Input: part model. Units: mm. Frame: model coordinates. Face numbers are marked on the shaded views. A direction names the side the tool comes from. Coordinates: 2 decimals unless noted, no trailing zeros. Order: outer loops, then holes, each group sorted by start corner. A loop starts at its lowest first (then second) coordinate and runs counter-clockwise, first axis right, second up. Notation, with made-up numbers: M 88,41.5 L 132,41.5 A18 ccw 132,61.5 Z; hole C -35,76 d7. An arc over 180 degrees is marked long. Answer in a Markdown table with one row per item.
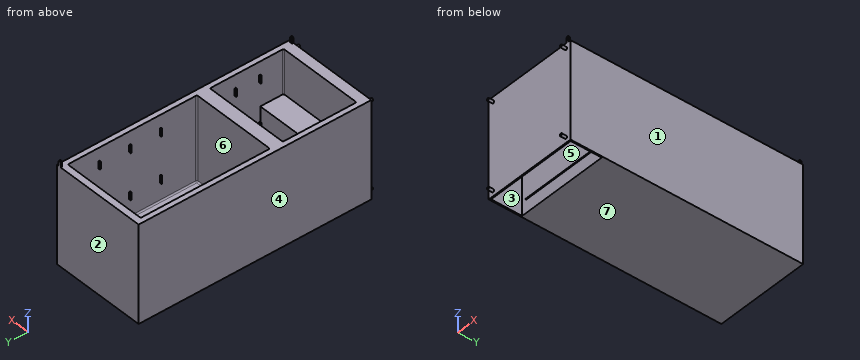
from build123d import *
from OCP.BRepFilletAPI import BRepFilletAPI_MakeChamfer

# Parameters (mm, degrees)
ESBO_O1_W                = 740
ESBO_O1_H                = 750
RESSALTO_EXTRUS_O1_DEPTH = 1800
ESBO_O5_W                = 660
ESBO_O5_H                = 1000
ESBO_O5_H_2              = 570
CORTE_EXTRUS_O1_DEPTH    = 650
FILETE1_R                = 10
ESBO_O7_R                = 10
RESSALTO_EXTRUS_O3_DEPTH = 40
ESBO_O10_W               = 55
ESBO_O10_H               = 10
RESSALTO_EXTRUS_O4_DEPTH = 15
ESBO_O14_W               = 55
ESBO_O14_H               = 10
RESSALTO_EXTRUS_O5_DEPTH = 15
CHANFRO1_SIZE            = 5
CHANFRO1_SIZE2           = 5.958767963
RESSALTO_EXTRUS_O6_DEPTH = 10
ESBO_O18_R               = 5
CORTE_EXTRUS_O2_DEPTH    = 5
ESBO_O19_W               = 720
ESBO_O19_H               = 240
CORTE_EXTRUS_O5_DEPTH    = 400
RESSALTO_EXTRUS_O8_REACH = 2073.835


with BuildPart() as part:
    # Esboço1 → Ressalto-extrusão1 (new body)
    with BuildSketch(Plane(origin=(0, 0, 0), x_dir=(1, 0, 0), z_dir=(0, 1, 0))):
        with Locations((370, 375)):
            Rectangle(ESBO_O1_W, ESBO_O1_H)
    extrude(amount=RESSALTO_EXTRUS_O1_DEPTH)

    # Esboço5 → Corte-extrusão1 (cut)
    with BuildSketch(Plane.XY):
        with Locations((370, 1250)):
            Rectangle(ESBO_O5_W, ESBO_O5_H)
        with Locations((370, 365)):
            Rectangle(ESBO_O5_W, ESBO_O5_H_2)
    extrude(amount=-CORTE_EXTRUS_O1_DEPTH, mode=Mode.SUBTRACT)

    # Filete1
    filete1_edges = [part.edges().sort_by_distance(p)[0] for p in [
        (40, 1250, -650),
        (40, 750, -325),
        (370, 1750, -650),
        (40, 1750, -325),
        (700, 1250, -650),
        (700, 1750, -325),
        (370, 750, -650),
        (700, 750, -325),
        (40, 365, -650),
        (40, 80, -325),
        (370, 650, -650),
        (40, 650, -325),
        (700, 365, -650),
        (700, 650, -325),
        (370, 80, -650),
        (700, 80, -325),
    ]]
    fillet(filete1_edges, radius=FILETE1_R)

    # Esboço7 → Ressalto-extrusão3 (add)
    with BuildSketch(Plane.XZ):
        with Locations(Location((40, -40, 0), (0, 0, 270))):
            Circle(ESBO_O7_R)
        with Locations(Location((700, -40, 0), (0, 0, 270))):
            Circle(ESBO_O7_R)
        with Locations(Location((700, -710, 0), (0, 0, 270))):
            Circle(ESBO_O7_R)
        with Locations(Location((40, -710, 0), (0, 0, 270))):
            Circle(ESBO_O7_R)
    extrude(amount=RESSALTO_EXTRUS_O3_DEPTH)

    # Esboço10 → Ressalto-extrusão4 (add)
    with BuildSketch(Plane(origin=(40, 0, 0), x_dir=(0, 0, -1), z_dir=(1, 0, 0))):
        with Locations((127.5, 1507.5)):
            Rectangle(ESBO_O10_W, ESBO_O10_H)
        with Locations((482.5, 1507.5)):
            Rectangle(ESBO_O10_W, ESBO_O10_H)
        with Locations((482.5, 1270)):
            Rectangle(ESBO_O10_W, ESBO_O10_H)
        with Locations((482.5, 1032.5)):
            Rectangle(ESBO_O10_W, ESBO_O10_H)
        with Locations((127.5, 1270)):
            Rectangle(ESBO_O10_W, ESBO_O10_H)
        with Locations((127.5, 1032.5)):
            Rectangle(ESBO_O10_W, ESBO_O10_H)
    ressalto_extrus_o4 = extrude(amount=RESSALTO_EXTRUS_O4_DEPTH)

    # Espelhar4: Ressalto-extrusão4 across plane
    add(ressalto_extrus_o4.mirror(Plane(origin=(370, 0, 0), x_dir=(0, 0, 1), z_dir=(1, 0, 0))))

    # Esboço14 → Ressalto-extrusão5 (add)
    with BuildSketch(Plane(origin=(40, 0, 0), x_dir=(0, 0, -1), z_dir=(1, 0, 0))):
        with Locations((127.5, 455)):
            Rectangle(ESBO_O14_W, ESBO_O14_H)
        with Locations((482.5, 455)):
            Rectangle(ESBO_O14_W, ESBO_O14_H)
        with Locations((482.5, 265)):
            Rectangle(ESBO_O14_W, ESBO_O14_H)
        with Locations((127.5, 265)):
            Rectangle(ESBO_O14_W, ESBO_O14_H)
    ressalto_extrus_o5 = extrude(amount=RESSALTO_EXTRUS_O5_DEPTH)

    # Espelhar5: Ressalto-extrusão5 across plane
    add(ressalto_extrus_o5.mirror(Plane(origin=(370, 0, 0), x_dir=(0, 0, 1), z_dir=(1, 0, 0))))

    # Chanfro1: one chamfer whose edges measure the first distance from different faces: ONE call of the kernel's chamfer builder (chamfer() names one face for all edges)
    chanfro1_edges_1 = [part.edges().sort_by_distance(p)[0] for p in [
        (55, 1502.5, -127.5),
    ]]
    chanfro1_side_1 = [part.faces().sort_by_distance(p)[0] for p in [
        (55, 1507.5, -127.5),
    ]]
    chanfro1_edges_2 = [part.edges().sort_by_distance(p)[0] for p in [
        (55, 1502.5, -482.5),
    ]]
    chanfro1_side_2 = [part.faces().sort_by_distance(p)[0] for p in [
        (55, 1507.5, -482.5),
    ]]
    chanfro1_edges_3 = [part.edges().sort_by_distance(p)[0] for p in [
        (55, 1265, -482.5),
    ]]
    chanfro1_side_3 = [part.faces().sort_by_distance(p)[0] for p in [
        (55, 1270, -482.5),
    ]]
    chanfro1_edges_4 = [part.edges().sort_by_distance(p)[0] for p in [
        (55, 1027.5, -482.5),
    ]]
    chanfro1_side_4 = [part.faces().sort_by_distance(p)[0] for p in [
        (55, 1032.5, -482.5),
    ]]
    chanfro1_edges_5 = [part.edges().sort_by_distance(p)[0] for p in [
        (55, 1265, -127.5),
    ]]
    chanfro1_side_5 = [part.faces().sort_by_distance(p)[0] for p in [
        (55, 1270, -127.5),
    ]]
    chanfro1_edges_6 = [part.edges().sort_by_distance(p)[0] for p in [
        (55, 1027.5, -127.5),
    ]]
    chanfro1_side_6 = [part.faces().sort_by_distance(p)[0] for p in [
        (55, 1032.5, -127.5),
    ]]
    chanfro1_edges_7 = [part.edges().sort_by_distance(p)[0] for p in [
        (685, 1502.5, -127.5),
    ]]
    chanfro1_side_7 = [part.faces().sort_by_distance(p)[0] for p in [
        (692.5, 1502.5, -127.5),
    ]]
    chanfro1_edges_8 = [part.edges().sort_by_distance(p)[0] for p in [
        (685, 1502.5, -482.5),
    ]]
    chanfro1_side_8 = [part.faces().sort_by_distance(p)[0] for p in [
        (692.5, 1502.5, -482.5),
    ]]
    chanfro1_edges_9 = [part.edges().sort_by_distance(p)[0] for p in [
        (685, 1265, -482.5),
    ]]
    chanfro1_side_9 = [part.faces().sort_by_distance(p)[0] for p in [
        (692.5, 1265, -482.5),
    ]]
    chanfro1_edges_10 = [part.edges().sort_by_distance(p)[0] for p in [
        (685, 1027.5, -482.5),
    ]]
    chanfro1_side_10 = [part.faces().sort_by_distance(p)[0] for p in [
        (692.5, 1027.5, -482.5),
    ]]
    chanfro1_edges_11 = [part.edges().sort_by_distance(p)[0] for p in [
        (685, 1265, -127.5),
    ]]
    chanfro1_side_11 = [part.faces().sort_by_distance(p)[0] for p in [
        (692.5, 1265, -127.5),
    ]]
    chanfro1_edges_12 = [part.edges().sort_by_distance(p)[0] for p in [
        (685, 1027.5, -127.5),
    ]]
    chanfro1_side_12 = [part.faces().sort_by_distance(p)[0] for p in [
        (692.5, 1027.5, -127.5),
    ]]
    chanfro1_edges_13 = [part.edges().sort_by_distance(p)[0] for p in [
        (55, 450, -127.5),
    ]]
    chanfro1_side_13 = [part.faces().sort_by_distance(p)[0] for p in [
        (55, 455, -127.5),
    ]]
    chanfro1_edges_14 = [part.edges().sort_by_distance(p)[0] for p in [
        (55, 450, -482.5),
    ]]
    chanfro1_side_14 = [part.faces().sort_by_distance(p)[0] for p in [
        (55, 455, -482.5),
    ]]
    chanfro1_edges_15 = [part.edges().sort_by_distance(p)[0] for p in [
        (55, 260, -482.5),
    ]]
    chanfro1_side_15 = [part.faces().sort_by_distance(p)[0] for p in [
        (55, 265, -482.5),
    ]]
    chanfro1_edges_16 = [part.edges().sort_by_distance(p)[0] for p in [
        (55, 260, -127.5),
    ]]
    chanfro1_side_16 = [part.faces().sort_by_distance(p)[0] for p in [
        (55, 265, -127.5),
    ]]
    chanfro1_edges_17 = [part.edges().sort_by_distance(p)[0] for p in [
        (685, 450, -127.5),
    ]]
    chanfro1_side_17 = [part.faces().sort_by_distance(p)[0] for p in [
        (692.5, 450, -127.5),
    ]]
    chanfro1_edges_18 = [part.edges().sort_by_distance(p)[0] for p in [
        (685, 450, -482.5),
    ]]
    chanfro1_side_18 = [part.faces().sort_by_distance(p)[0] for p in [
        (692.5, 450, -482.5),
    ]]
    chanfro1_edges_19 = [part.edges().sort_by_distance(p)[0] for p in [
        (685, 260, -482.5),
    ]]
    chanfro1_side_19 = [part.faces().sort_by_distance(p)[0] for p in [
        (692.5, 260, -482.5),
    ]]
    chanfro1_edges_20 = [part.edges().sort_by_distance(p)[0] for p in [
        (685, 260, -127.5),
    ]]
    chanfro1_side_20 = [part.faces().sort_by_distance(p)[0] for p in [
        (692.5, 260, -127.5),
    ]]
    chanfro1 = BRepFilletAPI_MakeChamfer(part.part.solid().wrapped)
    for e in chanfro1_edges_1:
        chanfro1.Add(CHANFRO1_SIZE, CHANFRO1_SIZE2, e.wrapped, chanfro1_side_1[0].wrapped)  # the first distance lies on this face
    for e in chanfro1_edges_2:
        chanfro1.Add(CHANFRO1_SIZE, CHANFRO1_SIZE2, e.wrapped, chanfro1_side_2[0].wrapped)  # the first distance lies on this face
    for e in chanfro1_edges_3:
        chanfro1.Add(CHANFRO1_SIZE, CHANFRO1_SIZE2, e.wrapped, chanfro1_side_3[0].wrapped)  # the first distance lies on this face
    for e in chanfro1_edges_4:
        chanfro1.Add(CHANFRO1_SIZE, CHANFRO1_SIZE2, e.wrapped, chanfro1_side_4[0].wrapped)  # the first distance lies on this face
    for e in chanfro1_edges_5:
        chanfro1.Add(CHANFRO1_SIZE, CHANFRO1_SIZE2, e.wrapped, chanfro1_side_5[0].wrapped)  # the first distance lies on this face
    for e in chanfro1_edges_6:
        chanfro1.Add(CHANFRO1_SIZE, CHANFRO1_SIZE2, e.wrapped, chanfro1_side_6[0].wrapped)  # the first distance lies on this face
    for e in chanfro1_edges_7:
        chanfro1.Add(CHANFRO1_SIZE, CHANFRO1_SIZE2, e.wrapped, chanfro1_side_7[0].wrapped)  # the first distance lies on this face
    for e in chanfro1_edges_8:
        chanfro1.Add(CHANFRO1_SIZE, CHANFRO1_SIZE2, e.wrapped, chanfro1_side_8[0].wrapped)  # the first distance lies on this face
    for e in chanfro1_edges_9:
        chanfro1.Add(CHANFRO1_SIZE, CHANFRO1_SIZE2, e.wrapped, chanfro1_side_9[0].wrapped)  # the first distance lies on this face
    for e in chanfro1_edges_10:
        chanfro1.Add(CHANFRO1_SIZE, CHANFRO1_SIZE2, e.wrapped, chanfro1_side_10[0].wrapped)  # the first distance lies on this face
    for e in chanfro1_edges_11:
        chanfro1.Add(CHANFRO1_SIZE, CHANFRO1_SIZE2, e.wrapped, chanfro1_side_11[0].wrapped)  # the first distance lies on this face
    for e in chanfro1_edges_12:
        chanfro1.Add(CHANFRO1_SIZE, CHANFRO1_SIZE2, e.wrapped, chanfro1_side_12[0].wrapped)  # the first distance lies on this face
    for e in chanfro1_edges_13:
        chanfro1.Add(CHANFRO1_SIZE, CHANFRO1_SIZE2, e.wrapped, chanfro1_side_13[0].wrapped)  # the first distance lies on this face
    for e in chanfro1_edges_14:
        chanfro1.Add(CHANFRO1_SIZE, CHANFRO1_SIZE2, e.wrapped, chanfro1_side_14[0].wrapped)  # the first distance lies on this face
    for e in chanfro1_edges_15:
        chanfro1.Add(CHANFRO1_SIZE, CHANFRO1_SIZE2, e.wrapped, chanfro1_side_15[0].wrapped)  # the first distance lies on this face
    for e in chanfro1_edges_16:
        chanfro1.Add(CHANFRO1_SIZE, CHANFRO1_SIZE2, e.wrapped, chanfro1_side_16[0].wrapped)  # the first distance lies on this face
    for e in chanfro1_edges_17:
        chanfro1.Add(CHANFRO1_SIZE, CHANFRO1_SIZE2, e.wrapped, chanfro1_side_17[0].wrapped)  # the first distance lies on this face
    for e in chanfro1_edges_18:
        chanfro1.Add(CHANFRO1_SIZE, CHANFRO1_SIZE2, e.wrapped, chanfro1_side_18[0].wrapped)  # the first distance lies on this face
    for e in chanfro1_edges_19:
        chanfro1.Add(CHANFRO1_SIZE, CHANFRO1_SIZE2, e.wrapped, chanfro1_side_19[0].wrapped)  # the first distance lies on this face
    for e in chanfro1_edges_20:
        chanfro1.Add(CHANFRO1_SIZE, CHANFRO1_SIZE2, e.wrapped, chanfro1_side_20[0].wrapped)  # the first distance lies on this face
    add(Compound.cast(chanfro1.Shape()), mode=Mode.REPLACE)

    # Esboço17 → Ressalto-extrusão6 (add)
    with BuildSketch(Plane(origin=(0, 1800, 0), x_dir=(1, 0, 0), z_dir=(0, 1, 0))):
        with BuildLine():
            Line((703.893019461, 0), (723.893019461, 0))
            Line((723.893019461, 0), (723.893019461, -35))
            ThreePointArc((723.893019461, -35), (713.893019461, -45), (703.893019461, -35))
            Line((703.893019461, -35), (703.893019461, 0))
        make_face()
    ressalto_extrus_o6 = extrude(amount=-RESSALTO_EXTRUS_O6_DEPTH)

    # Esboço18 → Corte-extrusão2 (cut)
    with BuildSketch(Plane.XZ.offset(-1790)):
        with Locations(Location((713.893019461, 35, 0), (0, 0, 270))):
            Circle(ESBO_O18_R)
    corte_extrus_o2 = extrude(amount=-CORTE_EXTRUS_O2_DEPTH, mode=Mode.SUBTRACT)

    # Espelhar6: Ressalto-extrusão6, Corte-extrusão2 across plane
    add(ressalto_extrus_o6.mirror(Plane.ZX.offset(900)))
    add(corte_extrus_o2.mirror(Plane.ZX.offset(900)), mode=Mode.SUBTRACT)

    # Esboço19 → Corte-extrusão5 (cut)
    with BuildSketch(Plane(origin=(0, 0, -750), x_dir=(-1, 0, 0), z_dir=(0, 0, -1))):
        with Locations((-370, 130)):
            Rectangle(ESBO_O19_W, ESBO_O19_H)
    extrude(amount=-CORTE_EXTRUS_O5_DEPTH, mode=Mode.SUBTRACT)

    # Esboço21 → Ressalto-extrusão8 (add, up to next)
    with BuildSketch(Plane.ZY.offset(-700), mode=Mode.PRIVATE) as ressalto_extrus_o8_sk1:
        Polygon((-640, 250), (-350, 250), (-350, 0), (-340, 0), (-340, 260), (-640, 260), align=None)
    ressalto_extrus_o8_tool1 = extrude(ressalto_extrus_o8_sk1.sketch, amount=RESSALTO_EXTRUS_O8_REACH, mode=Mode.PRIVATE) - part.part
    add(ressalto_extrus_o8_tool1.solids().sort_by_distance((700, 253.969887, -495))[0])


solid = part.part
1) Contact query for flat-ended pins moving along their axis: pin 1 (11 mm diameter, centred on x = 696, z = -131, fed in from -Y); pin 2 (8 mm diameter, centred on x = 50, y = 1506, fed in from +Z); pin 3 (3 mm diameter, centred on x = 368, y = 355, fed in from +Z). Output: stop coordinate, or through.
Resolved:
| item | result |
|---|---|
| pin 1 | stops at y = 0 |
| pin 2 | stops at z = -100 |
| pin 3 | stops at z = -650 |
2) Material intervals for probe 1 along Y at (x, z) = (180, -78); probe 2 along Y at (x, z) = (65.5, -596.5); probe 3 along X at (y, z) = (339, -89), sorted ascending.
Resolved:
| item | result |
|---|---|
| probe 1 | y = 0 to 80, 650 to 750, 1750 to 1800 |
| probe 2 | y = 0 to 10, 250 to 260, 650 to 750, 1750 to 1800 |
| probe 3 | x = 0 to 40, 700 to 740 |
3) Reachability of the marked faces 5, 6 and 7 from +Z, -Z, +X, -X, +Y, -Y: full face, straight path, thin tool, end or side. Return the list, or none.
Resolved:
| item | result |
|---|---|
| face 5 | -Z |
| face 6 | +Z |
| face 7 | -Z, +X, -X, +Y, -Y |
4) Mould query, pull axis X, two halves, no side actions, for the marked faces 1, 2, 3 and 4. Classes: +X half, -X half, draft (parallel to the pull), parting line (faces both ways), or undercut.
Resolved:
| item | result |
|---|---|
| face 1 | +X half |
| face 2 | draft |
| face 3 | undercut |
| face 4 | -X half |
5) Cut plane C-C, the plane z = -399. Output: boundary loops of the cut face in (x, y).
Resolved:
| item | result |
|---|---|
| outline | M 0,0 L 740,0 L 740,1800 L 0,1800 Z; hole M 10,10 L 730,10 L 730,250 L 10,250 Z; hole M 40,260 L 700,260 L 700,640 A10 ccw 690,650 L 50,650 A10 ccw 40,640 Z; hole M 40,760 A10 ccw 50,750 L 690,750 A10 ccw 700,760 L 700,1740 A10 ccw 690,1750 L 50,1750 A10 ccw 40,1740 Z |
6) Cut plane A-A, the plane x = 480. Output: boundary loops of the cut face in (y, z), and give its area (3 significant figures).
Resolved:
| item | result |
|---|---|
| outline | M 0,-750 L 10,-750 L 10,-350 L 250,-350 L 250,-640 L 260,-640 L 260,-340 L 80,-340 L 80,0 L 0,0 Z; M 250,-750 L 1800,-750 L 1800,0 L 1750,0 L 1750,-640 A10 cw 1740,-650 L 760,-650 A10 cw 750,-640 L 750,0 L 650,0 L 650,-640 A10 cw 640,-650 L 250,-650 Z |
| area | 289,000 mm2 |
7) Cut plane D-D, the plane y = 399.5. Output: boundary loops of the cut face in (x, z), and give its area (3 significant figures).
Resolved:
| item | result |
|---|---|
| outline | M 0,-750 L 740,-750 L 740,0 L 700,0 L 700,-640 A10 cw 690,-650 L 50,-650 A10 cw 40,-640 L 40,0 L 0,0 Z |
| area | 126,000 mm2 |
8) Cut plane B-B, the plane z = -218. Output: boundary loops of the cut face in (x, y), and give its area (3 significant figures).
Resolved:
| item | result |
|---|---|
| outline | M 0,0 L 740,0 L 740,1800 L 0,1800 Z; hole M 40,90 A10 ccw 50,80 L 690,80 A10 ccw 700,90 L 700,640 A10 ccw 690,650 L 50,650 A10 ccw 40,640 Z; hole M 40,760 A10 ccw 50,750 L 690,750 A10 ccw 700,760 L 700,1740 A10 ccw 690,1750 L 50,1750 A10 ccw 40,1740 Z |
| area | 296,000 mm2 |
